```python
from build123d import *

# Parameters (mm, degrees)
SKETCH_1_R          = 2.1
EXTRUDE_1_DEPTH     = 1.6
SKETCH_2_W          = 15.831082037
SKETCH_2_H          = 12.45501042
SKETCH_2_W_2        = 15.680188414
SKETCH_2_H_2        = 13.80676649
SKETCH_2_H_3        = 4.979489554
EXTRUDE_2_DEPTH     = 10
SKETCH_4_W          = 11.752987814
SKETCH_4_H          = 3.899349988
SKETCH_4_W_2        = 9.690175718
SKETCH_4_H_2        = 1.018486937
SKETCH_4_W_3        = 11.742918051
SKETCH_4_H_3        = 3.771361158
SKETCH_4_H_4        = 0.81478955
CUT_EXTRUDE_1_DEPTH = 10
SKETCH_5_W          = 11.02482594
SKETCH_5_H          = 8.828308894
CUT_EXTRUDE_3_DEPTH = 10
SKETCH_6_W          = 3.67494198
SKETCH_6_H          = 8.448142483
SKETCH_6_W_2        = 0.887054961
SKETCH_6_H_2        = 7.054198973
CUT_EXTRUDE_4_DEPTH = 10
SKETCH_7_W          = 14.31905698
SKETCH_7_H          = 12.92692644
SKETCH_7_W_2        = 6.032565672
SKETCH_7_H_2        = 12.131423274
SKETCH_7_W_3        = 5.899981811
SKETCH_7_H_3        = 6.098857603
SKETCH_7_W_4        = 5.303354437
SKETCH_7_H_4        = 5.237062506
SKETCH_7_W_5        = 15.84377138
SKETCH_7_H_5        = 7.888739725
EXTRUDE_3_DEPTH     = 1
SKETCH_8_W          = 17.434777712
SKETCH_8_H          = 8.750534821
EXTRUDE_4_DEPTH     = 5
SKETCH_9_W          = 14.45164084
SKETCH_9_H          = 2.585385288
CUT_EXTRUDE_5_DEPTH = 5
SKETCH_10_W         = 7.345813671
SKETCH_10_H         = 9.262112889
EXTRUDE_5_DEPTH     = 3
SKETCH_11_W         = 7.769719093
SKETCH_11_H         = 1.711972004
CUT_EXTRUDE_6_DEPTH = 3


with BuildPart() as part:
    # 草图1 → 凸台-拉伸1 (new body)
    with BuildSketch(Plane(origin=(0, 0, 0), x_dir=(1, 0, 0), z_dir=(0, 1, 0))):
        with BuildLine():
            Line((-38, -28), (38, -28))
            ThreePointArc((38, -28), (41.181980515, -26.681980515), (42.5, -23.5))
            Line((42.5, -23.5), (42.5, 23.5))
            ThreePointArc((42.5, 23.5), (41.181980515, 26.681980515), (38, 28))
            Line((38, 28), (-38, 28))
            ThreePointArc((-38, 28), (-41.181980515, 26.681980515), (-42.5, 23.5))
            Line((-42.5, 23.5), (-42.5, -23.5))
            ThreePointArc((-42.5, -23.5), (-41.181980515, -26.681980515), (-38, -28))
        make_face()
        with Locations(Location((-38, 23.5, 0), (0, 0, 270))):
            Circle(SKETCH_1_R, mode=Mode.SUBTRACT)
        with Locations(Location((38, 23.5, 0), (0, 0, 270))):
            Circle(SKETCH_1_R, mode=Mode.SUBTRACT)
        with Locations(Location((38, -23.5, 0), (0, 0, 270))):
            Circle(SKETCH_1_R, mode=Mode.SUBTRACT)
        with Locations(Location((-38, -23.5, 0), (0, 0, 270))):
            Circle(SKETCH_1_R, mode=Mode.SUBTRACT)
    extrude(amount=EXTRUDE_1_DEPTH)

    # 草图2 → 凸台-拉伸2 (add)
    with BuildSketch(Plane(origin=(0, 1.6, 0), x_dir=(1, 0, 0), z_dir=(0, 1, 0))):
        with Locations((37.470005744, 4.267247856)):
            Rectangle(SKETCH_2_W, SKETCH_2_H)
        with Locations((37.394558932, -11.196205219)):
            Rectangle(SKETCH_2_W_2, SKETCH_2_H_2)
        with Locations((37.470005744, 16.077817111)):
            Rectangle(SKETCH_2_W, SKETCH_2_H_3)
    extrude(amount=EXTRUDE_2_DEPTH)

    # 草图4 → 切除-拉伸1 (cut)
    # profile 1 of 2: a face of its own
    with BuildSketch(Plane(origin=(45.234653139, 0, 0), x_dir=(0, 0, -1), z_dir=(1, 0, 0))):
        with Locations((-11.23099462, 9.288009883)):
            Rectangle(SKETCH_4_W, SKETCH_4_H)
        with Locations((-11.072577375, 9.826352979)):
            Rectangle(SKETCH_4_W_2, SKETCH_4_H_2, mode=Mode.SUBTRACT)
    # profile 2 of 2: a face of its own
    with BuildSketch(Plane(origin=(45.234653139, 0, 0), x_dir=(0, 0, -1), z_dir=(1, 0, 0))):
        with Locations((-11.236029502, 4.259569612)):
            Rectangle(SKETCH_4_W_3, SKETCH_4_H_3)
        with Locations((-11.072577375, 4.632069598)):
            Rectangle(SKETCH_4_W_2, SKETCH_4_H_4, mode=Mode.SUBTRACT)
    extrude(amount=-CUT_EXTRUDE_1_DEPTH, mode=Mode.SUBTRACT)

    # 草图5 → 切除-拉伸3 (cut)
    with BuildSketch(Plane(origin=(45.385546762, 0, 0), x_dir=(0, 0, -1), z_dir=(1, 0, 0))):
        with Locations((4.329673022, 6.294177297)):
            Rectangle(SKETCH_5_W, SKETCH_5_H)
    extrude(amount=-CUT_EXTRUDE_3_DEPTH, mode=Mode.SUBTRACT)

    # 草图6 → 切除-拉伸4 (cut)
    with BuildSketch(Plane(origin=(45.385546762, 0, 0), x_dir=(0, 0, -1), z_dir=(1, 0, 0))):
        with Locations((16.283794635, 6.399779078)):
            Rectangle(SKETCH_6_W, SKETCH_6_H)
        with Locations((15.523461812, 6.294177298)):
            Rectangle(SKETCH_6_W_2, SKETCH_6_H_2, mode=Mode.SUBTRACT)
    extrude(amount=-CUT_EXTRUDE_4_DEPTH, mode=Mode.SUBTRACT)

    # 草图7 → 凸台-拉伸3 (add)
    with BuildSketch(Plane(origin=(0, 1.6, 0), x_dir=(1, 0, 0), z_dir=(0, 1, 0))):
        with Locations((12.579817698, -0.729211235)):
            Rectangle(SKETCH_7_W, SKETCH_7_H)
        with Locations((-17.417280836, 0.994378957)):
            Rectangle(SKETCH_7_W_2, SKETCH_7_H_2)
        with Locations((-25.306020561, 14.153327154)):
            Rectangle(SKETCH_7_W_3, SKETCH_7_H_3)
        with Locations((20.004513911, 16.771858407)):
            Rectangle(SKETCH_7_W_4, SKETCH_7_H_4)
        with Locations((-20.93075315, -19.489827555)):
            Rectangle(SKETCH_7_W_5, SKETCH_7_H_5)
    extrude(amount=EXTRUDE_3_DEPTH)

    # 草图8 → 凸台-拉伸4 (add)
    with BuildSketch(Plane(origin=(0, 1.6, 0), x_dir=(1, 0, 0), z_dir=(0, 1, 0))):
        with Locations((-2.700472273, -25.129807113)):
            Rectangle(SKETCH_8_W, SKETCH_8_H)
    extrude(amount=EXTRUDE_4_DEPTH)

    # 草图9 → 切除-拉伸5 (cut)
    with BuildSketch(Plane.XY.offset(29.505074523)):
        Polygon((-11.417861129, 1.6), (-11.417861129, 2.627524922), (-10.390336207, 1.6), align=None)
        with Locations((-2.667326308, 3.920217566)):
            Rectangle(SKETCH_9_W, SKETCH_9_H)
        Polygon((6.016916583, 1.6), (6.016916583, 2.370567657), (5.192747103, 1.6), align=None)
    extrude(amount=-CUT_EXTRUDE_5_DEPTH, mode=Mode.SUBTRACT)

    # 草图10 → 凸台-拉伸5 (add)
    with BuildSketch(Plane(origin=(0, 1.6, 0), x_dir=(1, 0, 0), z_dir=(0, 1, 0))):
        with Locations((-41.156730333, 13.42606725)):
            Rectangle(SKETCH_10_W, SKETCH_10_H)
    extrude(amount=EXTRUDE_5_DEPTH)

    # 草图11 → 切除-拉伸6 (cut)
    with BuildSketch(Plane.ZY.offset(44.829637168)):
        with Locations((-13.398155788, 2.916901541)):
            Rectangle(SKETCH_11_W, SKETCH_11_H)
    extrude(amount=-CUT_EXTRUDE_6_DEPTH, mode=Mode.SUBTRACT)


solid = part.part
```
Source: CAD feature listing. Evaluate the final solid. Frame: model axes, mm. A direction names the side the tool comes from. Give positions to 0.01 mm unless a question says otherwise; leave off trailing zeros. Loops run counter-clockwise (first coordinate to the right, second up) from the corner with the lowest first, then second, coordinate; pieces in that order, holes last. Notation, with made-up numbers: (-26.5, 9) - (11.5, 9) arc R23 ccw to (11.5, 18) - close; hole circle Ø3 at (27, 79.25). An arc over 180 degrees is marked (long way). Use CSV: the item, a comma, the result in double quotes. Start each with the question number.
1. Draft query along Z for faces 1 (the flat face through (29.554, 7, 11)), 2 (the flat face through (40, 4, 5.365)), 3 (the cylindrical face through (-41.217, 0.789, 26.647)). Return one class per face: +Z half, -Z half, draft (parallel to the pull), parting line (faces both ways), or undercut.
2. Ray query, L1, parallel to X at y = 0.75, z = -23.5; L2, parallel to Y at x = 39, z = 14; L3, parallel to X at y = 5.75, z = 27.5. Return the intervals inside material, ascending.
3. Section B-B (z = 11.5). Output: boundary loops of the cut face in (x, y).
4. Pin query (flat end, axial travel): pin 1 (2 mm diameter, centred on y = 4, z = 27.5, fed in from +X); pin 2 (9.5 mm diameter, centred on x = -6, z = 24.5, fed in from +Y); pin 3 (10 mm diameter, centred on x = -3, z = 1.5, fed in from +Y). Return the tip coordinate at first contact, or that it passes through.
5. Reachability of faces 4 (the flat face through (45.235, 7, 11)), 5 (the flat face through (40, 6, 1.183)), 6 (the flat face through (-41, 3, -8.795)) from +Z, -Z, +X, -X, +Y, -Y: full face, straight path, thin tool, end or side. Return the list, or none.
6. Section C-C (x = 0). Output: boundary loops of the cut face in (y, z), then the cut area to 3 significant figures.
7. Section A-A (x = -27). Output: boundary loops of the cut face in (y, z), then the cut area to 3 significant figures.
Response:
1,face 1,"draft"
1,face 2,"undercut"
1,face 3,"+Z half"
2,L1,"-42.5 to -40.1, -35.9 to 35.9, 40.1 to 42.5"
2,L2,"0 to 2.37, 4.22 to 5.04, 6.15 to 7.34, 9.32 to 10.34, 11.24 to 11.6"
2,L3,"-11.42 to 6.02"
3,outline,"(-42.5, 0) - (42.5, 0) - (42.5, 1.6) - (45.23, 1.6) - (45.23, 2.37) - (35.23, 2.37) - (35.23, 4.22) - (45.23, 4.22) - (45.23, 5.04) - (35.23, 5.04) - (35.23, 6.15) - (45.23, 6.15) - (45.23, 7.34) - (35.23, 7.34) - (35.23, 9.32) - (45.23, 9.32) - (45.23, 10.34) - (35.23, 10.34) - (35.23, 11.24) - (45.23, 11.24) - (45.23, 11.6) - (29.55, 11.6) - (29.55, 1.6) - (-42.5, 1.6) - close"
4,pin 1,"x = 6.02"
4,pin 2,"y = 6.6"
4,pin 3,"y = 1.6"
5,face 4,"+Z, +X, +Y, -Y"
5,face 5,"+X"
5,face 6,"+Z, -X, +Y"
6,outline,"(0, -28) - (1.6, -28) - (1.6, 20.75) - (6.6, 20.75) - (6.6, 29.51) - (5.21, 29.51) - (5.21, 24.51) - (2.63, 24.51) - (2.63, 29.51) - (1.6, 29.51) - (1.6, 28) - (0, 28) - close"
6,area,"120 mm²"
7,outline,"(0, -28) - (1.6, -28) - (1.6, -17.2) - (2.6, -17.2) - (2.6, -11.1) - (1.6, -11.1) - (1.6, 15.55) - (2.6, 15.55) - (2.6, 23.43) - (1.6, 23.43) - (1.6, 28) - (0, 28) - close"
7,area,"104 mm²"
